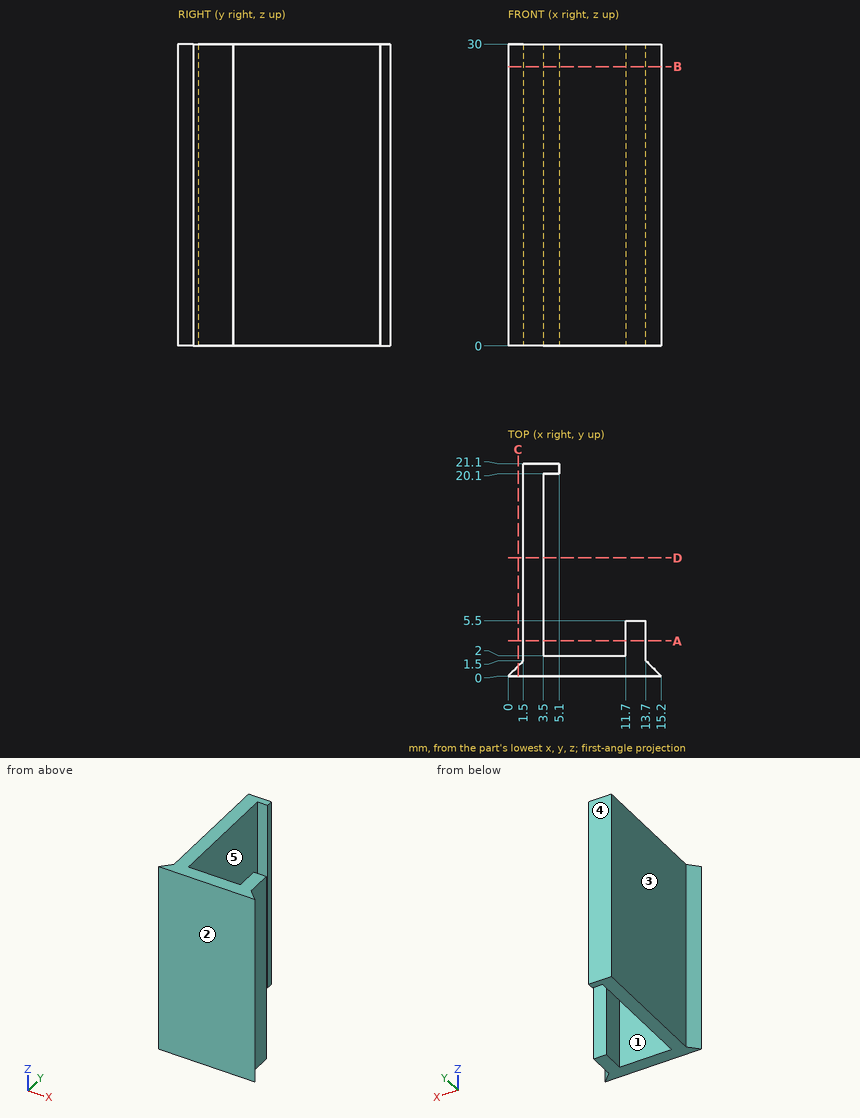
Can you work these out from the drawing? Everything is in mm from the part's minimum corner. A direction names the side the tool comes from. Coordinates: 2 decimals unless noted, no trailing zeros. Loops run counter-clockwise (first coordinate to the right, second up) from the corner with the lowest first, then second, coordinate; pieces in that order, holes last.
1. Imagine slicing it at B-B, the plane z = 27.75. Please give me the cut outline in (x, y).
2. I need wall thicknesses on L1, parallel to Y at x = 5, z = 14.25; L2, parallel to X at y = 2.75, z = 8; L3, parallel to X at y = 8, z = 3.25. Which ranges of each line are inside material? Lowest first, please.
3. Imagine slicing it at D-D, the plane y = 11.75. Please give me the cut outline in (x, z), and give its area (3 significant figures).
4. For the marked faces 4 and 5, which set-ups out of +Z, -Z, +X, -X, +Y, -Y let a thin tool reach every point of the face, with its end or its side?
5. If we mould it in two halves opening along X, with no side actions, what happens to the marked faces 1, 2 and 3? For each: pulls with the +X half, pulls with the -X half, needs draft (parallel to the pull), parting line crosses it, or undercut.
6. Imagine slicing it at C-C, the plane x = 1. Please give me the cut outline in (y, z), and give its area (3 significant figures).
7. For P1, Ø0.6, axis at x = 13, z = 12.5, coming from the +Y side; P2, Ø2, axis at y = 11.5, z = 25.5, coming from the +X side; P3, Ø1.1, axis at y = 20.5, z = 18, coming from the +X side, each with a flat end and sliding along its axis, tell me the tip position at first contact or that it passes through.
8. Imagine slicing it at A-A, the plane y = 3.5. Please give me the cut outline in (x, z), and give its area (3 significant figures).
Taken from the geometry:
1. outline: (0, 0) - (15.2, 0) - (13.7, 1.5) - (13.7, 5.5) - (11.7, 5.5) - (11.7, 2) - (3.5, 2) - (3.5, 20.1) - (5.1, 20.1) - (5.1, 21.1) - (1.5, 21.1) - (1.5, 1.5) - close
2. L1: y = 0 to 2, 20.1 to 21.1
2. L2: x = 1.5 to 3.5, 11.7 to 13.7
2. L3: x = 1.5 to 3.5
3. outline: (1.5, 0) - (3.5, 0) - (3.5, 30) - (1.5, 30) - close
3. area: 60.0 mm2
4. face 4: +Z, -Z, +X, -X, +Y
4. face 5: +Z, -Z
5. face 1: undercut
5. face 2: needs draft
5. face 3: pulls with the -X half
6. outline: (0, 0) - (1, 0) - (1, 30) - (0, 30) - close
6. area: 30.0 mm2
7. P1: stops at y = 5.5
7. P2: stops at x = 3.5
7. P3: stops at x = 5.1
8. outline: (1.5, 0) - (3.5, 0) - (3.5, 30) - (1.5, 30) - close; (11.7, 0) - (13.7, 0) - (13.7, 30) - (11.7, 30) - close
8. area: 120 mm2
